from build123d import *

# Parameters (mm, degrees)
F0_W     = 30
F0_H     = 15
F1_DEPTH = 50
F3_DEPTH = 30.001
F5_D     = 4


with BuildPart() as f1:
    # F0 (on Top) → F1 (new body)
    with BuildSketch(Plane.XY):
        with Locations((-23.119991, 11.377853)):
            Rectangle(F0_W, F0_H)
    extrude(amount=F1_DEPTH)

    # F2 (on face) → F3 (cut, through all)
    with BuildSketch(Plane(origin=(-38.119991, 0, 0), x_dir=(0, -1, 0), z_dir=(-1, 0, 0))):
        Polygon((-3.877853, 50), (-18.877853, 50), (-3.877853, 35), align=None)
        Polygon((-3.877853, 0), (-18.877853, 15), (-18.877853, 0), align=None)
    extrude(amount=-F3_DEPTH, mode=Mode.SUBTRACT)

    # F5 (through all)
    with Locations(Plane(origin=(0, 1.938926, -1.938926), x_dir=(-1, 0, 0), z_dir=(0, 0.707107, -0.707107))):
        with Locations((30.119991, 13.348658), (16.119991, 13.348658)):
            Hole(F5_D / 2)


solid = f1.part
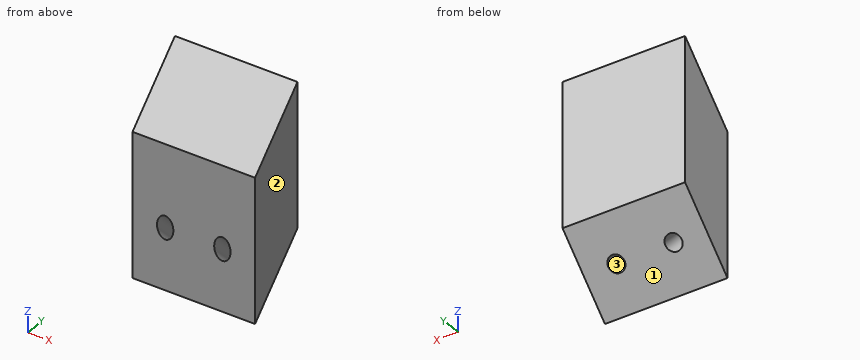
Verification items for the finished model (mm, model axes). Face numbers are marked on the shaded views. Give positions to 0.01 mm unless a question says otherwise; leave off trailing zeros. Write each loop counter-clockwise with the first axis right and the second up, starting at its lowest first coordinate (ties: lowest second). Pieces come first, ordered by that corner, then holes. Notation, with made-up numbers: M -5,30.25 L 0,30.25 A17 cw 0,40.25 Z; hole C 78,87 d6. An arc over 180 degrees is marked long. Write item = value, one per line.
(1) Go/stop test with flat-tipped pins: pin 1 Ø1.5 at (x, y) = (-26.5, 5.5) entering from +Z; pin 2 Ø2 at (x, y) = (-23, 14.5) entering from -Z; pin 3 Ø4 at (x, y) = (-29, 11.5) entering from +Z. Record where each tip stops, or that it passes through.
Found:
pin_1 = 37.37
pin_2 = 9.62
pin_3 = 44.62
(2) Sectioned sample at A-A (x = -15.5). Record the cut outline in (y, z), then the cut area to 3 significant figures.
Found:
outline = M 3.88,0 L 10.03,6.16 L 3.88,12.31 Z; M 3.88,17.69 L 12.72,8.84 L 18.88,15 L 18.88,50 L 3.88,35 Z
area = 485 mm2
(3) Sectioned sample at B-B (x = -31). Record the cut outline in (y, z).
Found:
outline = M 3.88,0 L 10.11,6.23 L 3.88,12.46 Z; M 3.88,17.54 L 12.65,8.77 L 18.88,15 L 18.88,50 L 3.88,35 Z
(4) Material ranges on line 1 (X direction, y = 7.5, z = 9); line 2 (Z direction, x = -16.5, y = 5.75); line 3 (Z direction, x = -35.5, y = 6.5), recorded low to high.
Found:
line_1 = -38.12 to -31.2, -29.04 to -17.2, -15.04 to -8.12
line_2 = 1.87 to 10.35, 15.9 to 36.87
line_3 = 2.62 to 37.62
(5) Draft check along Z on the marked faces 1, 2 and 3. Enter one of: released by +Z, released by -Z, zero draft, split by the parting line, or undercut.
Found:
face_1 = released by -Z
face_2 = zero draft
face_3 = undercut
(6) Sectioned sample at C-C (z = 44.5). Record the cut outline in (x, y).
Found:
outline = M -38.12,13.38 L -8.12,13.38 L -8.12,18.88 L -38.12,18.88 Z
(7) Sectioned sample at D-D (x = -11.5). Record the cut outline in (y, z), then the cut area to 3 significant figures.
Found:
outline = M 3.88,0 L 18.88,15 L 18.88,50 L 3.88,35 Z
area = 525 mm2
